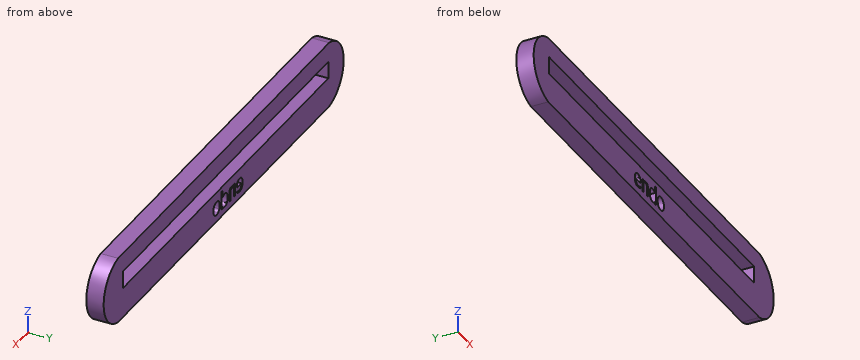
from build123d import *

# Parameters (mm, degrees)
F0_W     = 100
F0_H     = 4.4
F1_DEPTH = 4.4


with BuildPart() as f1:
    # F0 (on Front) → F1 (new body)
    with BuildSketch(Plane.XZ):
        with BuildLine():
            Line((52.5213778019, -35.3348962963), (-50.3410026431, -35.3348962963))
            ThreePointArc((-50.3410026431, -35.3348962963), (-57.4545573502, -43.799880892), (-50.3410026431, -52.2648654878))
            Line((-50.3410026431, -52.2648654878), (52.5213778019, -52.2648654878))
            ThreePointArc((52.5213778019, -52.2648654878), (59.5325622156, -43.799880892), (52.5213778019, -35.3348962963))
        make_face()
        with BuildLine():
            add(Edge.make_bspline(
                [(-6.0069680161, -50.4799766115), (-6.2456414194, -50.5306338237), (-6.5836808927, -50.5306338237)],
                knots=[0, 0, 0, 1, 1, 1], degree=2))
            add(Edge.make_bspline(
                [(-6.5836808927, -50.5306338237), (-7.3230813545, -50.5306338237), (-7.7512322148, -50.0795898002)],
                knots=[0, 0, 0, 1, 1, 1], degree=2))
            add(Edge.make_bspline(
                [(-7.7512322148, -50.0795898002), (-8.1793830751, -49.6285457767), (-8.1793830751, -48.8287463312)],
                knots=[0, 0, 0, 1, 1, 1], degree=2))
            add(Edge.make_bspline(
                [(-8.1793830751, -48.8287463312), (-8.1793830751, -48.0211534685), (-7.7819187952, -47.5462421046)],
                knots=[0, 0, 0, 1, 1, 1], degree=2))
            add(Edge.make_bspline(
                [(-7.7819187952, -47.5462421046), (-7.3844545154, -47.0713307408), (-6.7142206317, -47.0713307408)],
                knots=[0, 0, 0, 1, 1, 1], degree=2))
            add(Edge.make_bspline(
                [(-6.7142206317, -47.0713307408), (-6.08782472, -47.0713307408), (-5.7225082864, -47.4838947666)],
                knots=[0, 0, 0, 1, 1, 1], degree=2))
            add(Edge.make_bspline(
                [(-5.7225082864, -47.4838947666), (-5.3571918527, -47.8964587924), (-5.3571918527, -48.572537739)],
                knots=[0, 0, 0, 1, 1, 1], degree=2))
            Line((-5.3571918527, -48.572537739), (-5.3571918527, -48.8920678464))
            Line((-5.3571918527, -48.8920678464), (-7.6552757649, -48.8920678464))
            add(Edge.make_bspline(
                [(-7.6552757649, -48.8920678464), (-7.6396889304, -49.4794966718), (-7.3581517322, -49.7839270332)],
                knots=[0, 0, 0, 1, 1, 1], degree=2))
            add(Edge.make_bspline(
                [(-7.3581517322, -49.7839270332), (-7.0766145339, -50.0883573946), (-6.5651715267, -50.0883573946)],
                knots=[0, 0, 0, 1, 1, 1], degree=2))
            add(Edge.make_bspline(
                [(-6.5651715267, -50.0883573946), (-6.0264515592, -50.0883573946), (-5.5003958947, -49.8633224714)],
                knots=[0, 0, 0, 1, 1, 1], degree=2))
            Line((-5.5003958947, -49.8633224714), (-5.5003958947, -50.3143664949))
            add(Edge.make_bspline(
                [(-5.5003958947, -50.3143664949), (-5.7682946127, -50.4293193994), (-6.0069680161, -50.4799766115)],
                knots=[0, 0, 0, 1, 1, 1], degree=2))
        make_face(mode=Mode.SUBTRACT)
        with BuildLine():
            Line((-1.70597587, -50.4692606628), (-2.2115738142, -50.4692606628))
            Line((-2.2115738142, -50.4692606628), (-2.2115738142, -48.3104840839))
            add(Edge.make_bspline(
                [(-2.2115738142, -48.3104840839), (-2.2115738142, -47.9032780325), (-2.3971545626, -47.7021104497)],
                knots=[0, 0, 0, 1, 1, 1], degree=2))
            add(Edge.make_bspline(
                [(-2.3971545626, -47.7021104497), (-2.5827353109, -47.5009428669), (-2.9792254136, -47.5009428669)],
                knots=[0, 0, 0, 1, 1, 1], degree=2))
            add(Edge.make_bspline(
                [(-2.9792254136, -47.5009428669), (-3.5023585466, -47.5009428669), (-3.7459028358, -47.7839413308)],
                knots=[0, 0, 0, 1, 1, 1], degree=2))
            add(Edge.make_bspline(
                [(-3.7459028358, -47.7839413308), (-3.9894471249, -48.0669397948), (-3.9894471249, -48.7186643125)],
                knots=[0, 0, 0, 1, 1, 1], degree=2))
            Line((-3.9894471249, -48.7186643125), (-3.9894471249, -50.4692606628))
            Line((-3.9894471249, -50.4692606628), (-4.4950450691, -50.4692606628))
            Line((-4.4950450691, -50.4692606628), (-4.4950450691, -47.1327039017))
            Line((-4.4950450691, -47.1327039017), (-4.0839423091, -47.1327039017))
            Line((-4.0839423091, -47.1327039017), (-4.0021114279, -47.5895929881))
            Line((-4.0021114279, -47.5895929881), (-3.977756999, -47.5895929881))
            add(Edge.make_bspline(
                [(-3.977756999, -47.5895929881), (-3.821888654, -47.3431261675), (-3.5418127215, -47.2072284542)],
                knots=[0, 0, 0, 1, 1, 1], degree=2))
            add(Edge.make_bspline(
                [(-3.5418127215, -47.2072284542), (-3.261736789, -47.0713307408), (-2.9178522527, -47.0713307408)],
                knots=[0, 0, 0, 1, 1, 1], degree=2))
            add(Edge.make_bspline(
                [(-2.9178522527, -47.0713307408), (-2.3148365928, -47.0713307408), (-2.0104062314, -47.3621226221)],
                knots=[0, 0, 0, 1, 1, 1], degree=2))
            add(Edge.make_bspline(
                [(-2.0104062314, -47.3621226221), (-1.70597587, -47.6529145033), (-1.70597587, -48.2929488951)],
                knots=[0, 0, 0, 1, 1, 1], degree=2))
            Line((-1.70597587, -48.2929488951), (-1.70597587, -50.4692606628))
        make_face(mode=Mode.SUBTRACT)
        with BuildLine():
            Line((1.6695479773, -50.4692606628), (1.6023297535, -50.0221133479))
            Line((1.6023297535, -50.0221133479), (1.5750527932, -50.0221133479))
            add(Edge.make_bspline(
                [(1.5750527932, -50.0221133479), (1.225323194, -50.5306338237), (0.5278123499, -50.5306338237)],
                knots=[0, 0, 0, 1, 1, 1], degree=2))
            add(Edge.make_bspline(
                [(0.5278123499, -50.5306338237), (-0.1268346993, -50.5306338237), (-0.4906898672, -50.0829994202)],
                knots=[0, 0, 0, 1, 1, 1], degree=2))
            add(Edge.make_bspline(
                [(-0.4906898672, -50.0829994202), (-0.8545450352, -49.6353650168), (-0.8545450352, -48.8102369652)],
                knots=[0, 0, 0, 1, 1, 1], degree=2))
            add(Edge.make_bspline(
                [(-0.8545450352, -48.8102369652), (-0.8545450352, -47.9851089137), (-0.4892286015, -47.5282198273)],
                knots=[0, 0, 0, 1, 1, 1], degree=2))
            add(Edge.make_bspline(
                [(-0.4892286015, -47.5282198273), (-0.1239121678, -47.0713307408), (0.5278123499, -47.0713307408)],
                knots=[0, 0, 0, 1, 1, 1], degree=2))
            add(Edge.make_bspline(
                [(0.5278123499, -47.0713307408), (1.206813828, -47.0713307408), (1.5692077302, -47.5652385592)],
                knots=[0, 0, 0, 1, 1, 1], degree=2))
            Line((1.5692077302, -47.5652385592), (1.6091489936, -47.5652385592))
            Line((1.6091489936, -47.5652385592), (1.5877170962, -47.3246168015))
            Line((1.5877170962, -47.3246168015), (1.5750527932, -47.0898401068))
            Line((1.5750527932, -47.0898401068), (1.5750527932, -45.7318371506))
            Line((1.5750527932, -45.7318371506), (2.0806507374, -45.7318371506))
            Line((2.0806507374, -45.7318371506), (2.0806507374, -50.4692606628))
            Line((2.0806507374, -50.4692606628), (1.6695479773, -50.4692606628))
        make_face(mode=Mode.SUBTRACT)
        with Locations((0, -42.3694215596)):
            Rectangle(F0_W, F0_H, mode=Mode.SUBTRACT)
        with BuildLine():
            add(Edge.make_bspline(
                [(5.6193492585, -47.5374745102), (6.0319132843, -48.0036182796), (6.0319132843, -48.7975726622)],
                knots=[0, 0, 0, 1, 1, 1], degree=2))
            add(Edge.make_bspline(
                [(6.0319132843, -48.7975726622), (6.0319132843, -49.6139331194), (5.6212976128, -50.0722834715)],
                knots=[0, 0, 0, 1, 1, 1], degree=2))
            add(Edge.make_bspline(
                [(5.6212976128, -50.0722834715), (5.2106819413, -50.5306338237), (4.4858941369, -50.5306338237)],
                knots=[0, 0, 0, 1, 1, 1], degree=2))
            add(Edge.make_bspline(
                [(4.4858941369, -50.5306338237), (4.0377726449, -50.5306338237), (3.6909655771, -50.3202115578)],
                knots=[0, 0, 0, 1, 1, 1], degree=2))
            add(Edge.make_bspline(
                [(3.6909655771, -50.3202115578), (3.3441585094, -50.109789292), (3.155168141, -49.717195898)],
                knots=[0, 0, 0, 1, 1, 1], degree=2))
            add(Edge.make_bspline(
                [(3.155168141, -49.717195898), (2.9661777727, -49.3246025039), (2.9661777727, -48.7975726622)],
                knots=[0, 0, 0, 1, 1, 1], degree=2))
            add(Edge.make_bspline(
                [(2.9661777727, -48.7975726622), (2.9661777727, -47.9821863822), (3.3743580013, -47.5267585615)],
                knots=[0, 0, 0, 1, 1, 1], degree=2))
            add(Edge.make_bspline(
                [(3.3743580013, -47.5267585615), (3.7825382298, -47.0713307408), (4.5073260343, -47.0713307408)],
                knots=[0, 0, 0, 1, 1, 1], degree=2))
            add(Edge.make_bspline(
                [(4.5073260343, -47.0713307408), (5.2067852327, -47.0713307408), (5.6193492585, -47.5374745102)],
                knots=[0, 0, 0, 1, 1, 1], degree=2))
        make_face(mode=Mode.SUBTRACT)
    extrude(amount=F1_DEPTH)


solid = f1.part
Design review of the part built by this model. Coordinates are the model's own, in mm. Give positions to 0.01 mm unless a question says otherwise; leave off trailing zeros. Order: outer loops, then holes, each group sorted by start corner. A loop starts at its lowest first (then second) coordinate and runs counter-clockwise, first axis right, second up. Notation, with made-up numbers: (-38.75, -1) - (-11.75, -1) arc R18 ccw to (-11.75, 32) - close; hole circle Ø11 at (73.5, -3.5). An arc over 180 degrees is marked (long way). Use CSV: the item, a comma, the result in double quotes. Start each with the question number.
Q1. Take a section at A-A (x = -29). State the section outline as (y, z) points.
Q2. Take a section at C-C (y = -2.3). Count the separate pieces of the cut face and the enclosed holes in it, and give its area (3 significant figures).
Q3. For line 1 (Z direction, x = -24, y = -0.2); line 2 (X direction, y = -1.1, z = -43.25) (3 decimals); line 3 (Z direction, x = -6, y = -3.95), list the stretches that pass through material, from the lowest coordinate up.
Q4. For P1, Ø1.3, axis at y = -1.5, z = -43, coming from the -X side; P2, Ø1.3, axis at y = -2, z = -49, coming from the -X side; P3, Ø1.4, axis at y = -1.5, z = -50, coming from the -X side, all flat-tipped, find the tip position at first contact; note any pin that passes through.
Q5. Take a section at B-B (z = -43). State the section outline as (x, y) points.
Calculated:
1,outline,"(-4.4, -52.26) - (0, -52.26) - (0, -44.57) - (-4.4, -44.57) - close; (-4.4, -40.17) - (0, -40.17) - (0, -35.33) - (-4.4, -35.33) - close"
2,separate pieces,"1"
2,enclosed holes,"5"
2,area,"1,450 mm²"
3,line 1,"z = -52.26 to -44.57, -40.17 to -35.33"
3,line 2,"x = -57.437 to -50, 50 to 59.515"
3,line 3,"z = -52.26 to -50.48, -50.03 to -48.89, -47.25 to -44.57, -40.17 to -35.33"
4,P1,"stops at x = -57.45"
4,P2,"stops at x = -56.15"
4,P3,"stops at x = -55.46"
5,outline,"(-57.42, -4.4) - (-50, -4.4) - (-50, 0) - (-57.42, 0) - close; (50, -4.4) - (59.5, -4.4) - (59.5, 0) - (50, 0) - close"
